from build123d import *

# Parameters (mm, degrees)
SKETCH1_W           = 177.8
SKETCH1_H           = 177.8
SKETCH1_R           = 14.605
BOSS_EXTRUDE1_DEPTH = 3.175
SKETCH2_R           = 3.175
CUT_EXTRUDE1_DEPTH  = 4.175
SKETCH2_3_W         = 12.7
SKETCH2_3_H         = 109.98522628
BOSS_EXTRUDE2_DEPTH = 88.9
SKETCH3_R           = 6.35
CUT_EXTRUDE2_DEPTH  = 159.75


with BuildPart() as part:
    # Sketch1 → Boss-Extrude1 (new body)
    with BuildSketch(Plane.XY):
        Rectangle(SKETCH1_W, SKETCH1_H)
        Circle(SKETCH1_R, mode=Mode.SUBTRACT)
    extrude(amount=BOSS_EXTRUDE1_DEPTH)

    # Sketch2 → Cut-Extrude1 (cut, through all)
    with BuildSketch(Plane.XY.offset(3.175)):
        with Locations((-38.494829198, 22.225)):
            Circle(SKETCH2_R)
        with Locations((38.494829198, 22.225)):
            Circle(SKETCH2_R)
        with Locations((0, -44.45)):
            Circle(SKETCH2_R)
    extrude(amount=-CUT_EXTRUDE1_DEPTH, mode=Mode.SUBTRACT)

    # Sketch2_3 → Boss-Extrude2 (add)
    with BuildSketch(Plane.XY.offset(3.175)):
        with Locations((-63.5, 0)):
            Rectangle(SKETCH2_3_W, SKETCH2_3_H)
        with Locations((63.5, 0)):
            Rectangle(SKETCH2_3_W, SKETCH2_3_H)
    extrude(amount=BOSS_EXTRUDE2_DEPTH)

    # Sketch3 → Cut-Extrude2 (cut, through all)
    with BuildSketch(Plane.ZY.offset(69.85)):
        with BuildLine():
            Line((92.075, 54.99261314), (73.84861627, 54.99261314))
            ThreePointArc((73.84861627, 54.99261314), (87.399705252, 28.967173607), (92.075, 2.12e-07))
            Line((92.075, 2.12e-07), (92.075, 54.99261314))
        make_face()
        with BuildLine():
            ThreePointArc((92.075, 2.12e-07), (87.399705319, -28.967173406), (73.84861627, -54.99261314))
            Line((73.84861627, -54.99261314), (92.075, -54.99261314))
            Line((92.075, -54.99261314), (92.075, 2.12e-07))
        make_face()
        with Locations((73.025, 0)):
            Circle(SKETCH3_R)
    extrude(amount=-CUT_EXTRUDE2_DEPTH, mode=Mode.SUBTRACT)


solid = part.part
Geometry: final body of the model. Coordinates: model frame, mm. A direction names the side the tool comes from. Round coordinates to 2 decimals unless told otherwise and drop trailing zeros. Order: outer loops, then holes, each group sorted by start corner. A loop starts at its lowest first (then second) coordinate and runs counter-clockwise, first axis right, second up. Notation, with made-up numbers: (-1.75, 53) -> (28.25, 53) arc R24 ccw to (28.25, 92) -> close; hole circle Ø9 at (84, 21.25). An arc over 180 degrees is marked (long way). Put each result on its own line as item: value. Start each with the question number.
Q1. Section C-C on x = -37.5. Return the cut outline in (y, z) (3 decimals).
Q2. Reachability of faces 1 (the cylindrical face through (-0.4, -41.3, 1.6)), 2 (the flat face through (-69.85, -1, 47)), 3 (the flat face through (57.15, -1, 47)), 4 (the flat face through (63, -54.993, 38)), 5 (the flat face through (-64, 54.993, 38)) from +Z, -Z, +X, -X, +Y, -Y: full face, straight path, thin tool, end or side. Return the list, or none.
Q3. First-contact query: pin 1 (4 mm diameter, centred on x = -60, z = 11.5, fed in from +Y); pin 2 (4 mm diameter, centred on x = -63.5, z = 24.5, fed in from -Y); pin 3 (1.5 mm diameter, centred on y = 15.5, z = 38, fed in from -X). Flat tips, straight axial feed; report the tip coordinate or a pass-through.
Q4. Line query: probe 1 along X at (y, z) = (-24.5, 46); probe 2 along Z at (x, y) = (72, -41) (3 decimals); probe 3 along Z at (x, y) = (-69, -51). Output: solid intervals per line, ascending.
Q5. Pull-direction query (Y, two-part tool) for faces 6 (the flat face through (69.85, -1, 47)), 7 (the cylindrical face through (35.323, 22.365, 1.61)), 8 (the flat face through (-64, -54.993, 38)); classes: +Y half, -Y half, draft (parallel to the pull), parting line (faces both ways), or undercut.
Q6. Section A-A on z = 28.5. Return the cut outline in (x, y), and give its area (3 significant figures).
Q7. Section B-B on x = 0. Return the cut outline in (y, z) (3 decimals).
Q8. Section D-D on y = -44.45. Return the cut outline in (x, z) (3 decimals).
Ans:
1. outline: (-88.9, 0) -> (19.21, 0) -> (19.21, 3.175) -> (-88.9, 3.175) -> close; (25.24, 0) -> (88.9, 0) -> (88.9, 3.175) -> (25.24, 3.175) -> close
2. face 1: +Z, -Z
2. face 2: +Z, -X, +Y, -Y
2. face 3: +Z, +Y, -Y
2. face 4: +Z, +X, -X, -Y
2. face 5: +Z, +X, -X, +Y
3. pin 1: stops at y = 54.99
3. pin 2: stops at y = -54.99
3. pin 3: stops at x = -69.85
4. probe 1: x = -69.85 to -57.15, 57.15 to 69.85
4. probe 2: z = 0 to 3.175
4. probe 3: z = 0 to 76.66
5. face 6: draft
5. face 7: undercut
5. face 8: -Y half
6. outline: (-69.85, -54.99) -> (-57.15, -54.99) -> (-57.15, 54.99) -> (-69.85, 54.99) -> close; (57.15, -54.99) -> (69.85, -54.99) -> (69.85, 54.99) -> (57.15, 54.99) -> close
6. area: 2,790 mm2
7. outline: (-88.9, 0) -> (-47.625, 0) -> (-47.625, 3.175) -> (-88.9, 3.175) -> close; (-41.275, 0) -> (-14.605, 0) -> (-14.605, 3.175) -> (-41.275, 3.175) -> close; (14.605, 0) -> (88.9, 0) -> (88.9, 3.175) -> (14.605, 3.175) -> close
8. outline: (-88.9, 0) -> (-3.175, 0) -> (-3.175, 3.175) -> (-57.15, 3.175) -> (-57.15, 80.635) -> (-69.85, 80.635) -> (-69.85, 3.175) -> (-88.9, 3.175) -> close; (3.175, 0) -> (88.9, 0) -> (88.9, 3.175) -> (69.85, 3.175) -> (69.85, 80.635) -> (57.15, 80.635) -> (57.15, 3.175) -> (3.175, 3.175) -> close
